from build123d import *


with BuildPart() as f1:
    # F0 (on Top) → F1 (revolve)
    with BuildSketch(Plane.XY):
        with BuildLine():
            Line((256.921, 0), (0, 0))
            Line((0, 0), (0, -3.429))
            Line((0, -3.429), (257.57173, -3.429))
            Line((257.57173, -3.429), (267.802933, -13.660203))
            ThreePointArc((267.802933, -13.660203), (270.537497, -15.487381), (273.763136, -16.129))
            Line((273.763136, -16.129), (292.813136, -16.129))
            Line((292.813136, -16.129), (292.813136, -12.7))
            Line((292.813136, -12.7), (273.763136, -12.7))
            ThreePointArc((273.763136, -12.7), (271.849718, -12.319398), (270.227602, -11.235534))
            Line((270.227602, -11.235534), (260.456534, -1.464466))
            ThreePointArc((260.456534, -1.464466), (258.834417, -0.380602), (256.921, 0))
        make_face()
    revolve(axis=Axis((0, -1.7145, 0), (0, -1, 0)))


solid = f1.part
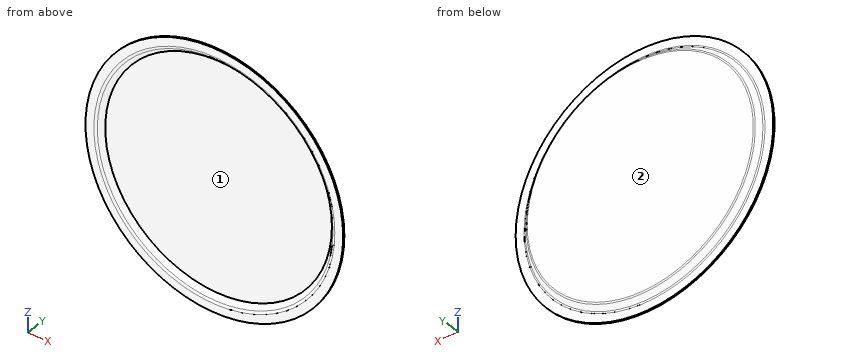
The model under review builds one solid part; all positions refer to its coordinate system, in mm. Face numbers are marked on the shaded views. Round coordinates to 2 decimals unless told otherwise and drop trailing zeros. Write each loop counter-clockwise with the first axis right and the second up, starting at its lowest first coordinate (ties: lowest second). Pieces come first, ordered by that corner, then holes. Notation, with made-up numbers: M 4.5,14.25 L 63.5,14.25 A20 ccw 63.5,37.25 Z; hole C -34,2.5 d2. An arc over 180 degrees is marked long. Use a Markdown table: item, result. Add a question column.
Q1. We need section B-B, the plane z = 0. State the section outline as (x, y) points, plus the area to 3 significant figures.
Q2. We need section C-C, the plane y = -7.5. State the section outline as (x, z) points, plus the area to 3 significant figures.
Q3. The part is to be moulded in two halves that separate along Z. For the marked faces 1 and 2, say which applies: pulls with the +Z half, pulls with the -Z half, needs draft (parallel to the pull), parting line crosses it, or undercut.
Q4. Insertion check: pin 1 (6 mm diameter, centred on x = -176, y = -13, fed in from +Z); pin 2 (3 mm diameter, centred on x = 206, z = -75.5, fed in from -Y); pin 3 (6 mm diameter, centred on y = -6.5, z = -225, fed in from +X). Each pin has a flat end and moves straight along its axis. Give the tip position at first contact, or say it passes through.
Q5. We need section A-A, the plane x = 0. State the section outline as (y, z) points, plus the area to 3 significant figures.
Q6. To check wall thickness, follow line 1 (Z direction, x = 15.5, y = -14.5); line 2 (X direction, y = -15.5, z = -43); line 3 (X direction, y = -3.5, z = -223). State the ranges of each line that lie inside material, in increasing order.
Findings below:
| question | item | result |
|---|---|---|
| 1 | outline | M -292.81,-16.13 L -273.76,-16.13 A8.43 ccw -267.8,-13.66 L -257.57,-3.43 L 257.57,-3.43 L 267.8,-13.66 A8.43 ccw 273.76,-16.13 L 292.81,-16.13 L 292.81,-12.7 L 273.76,-12.7 A5 cw 270.23,-11.24 L 260.46,-1.46 A5 ccw 256.92,0 L -256.92,0 A5 ccw -260.46,-1.46 L -270.23,-11.24 A5 cw -273.76,-12.7 L -292.81,-12.7 Z |
| 1 | area | 2,040 mm² |
| 2 | outline | C 0,0 d532.98; hole C 0,0 d523.29 |
| 2 | area | 8,050 mm² |
| 3 | face 1 | undercut |
| 3 | face 2 | needs draft |
| 4 | pin 1 | stops at z = 236.24 |
| 4 | pin 2 | stops at y = -3.43 |
| 4 | pin 3 | stops at x = 148.16 |
| 5 | outline | M -16.13,-292.81 L -12.7,-292.81 L -12.7,-273.76 A5 cw -11.24,-270.23 L -1.46,-260.46 A5 ccw 0,-256.92 L 0,256.92 A5 ccw -1.46,260.46 L -11.24,270.23 A5 cw -12.7,273.76 L -12.7,292.81 L -16.13,292.81 L -16.13,273.76 A8.43 ccw -13.66,267.8 L -3.43,257.57 L -3.43,-257.57 L -13.66,-267.8 A8.43 ccw -16.13,-273.76 Z |
| 5 | area | 2,040 mm² |
| 6 | line 1 | z = -292.4 to -268.34, 268.34 to 292.4 |
| 6 | line 2 | x = -289.64 to -267.13, 267.13 to 289.64 |
| 6 | line 3 | x = -138.47 to -129.04, 129.04 to 138.47 |
